Drawing for the job (mm, zero at the part's lowest x, y, z). A direction names the side the tool comes from. Give positions to 0.01 mm unless a question says otherwise; leave off trailing zeros. Order: outer loops, then holes, each group sorted by start corner. A loop starts at its lowest first (then second) coordinate and runs counter-clockwise, first axis right, second up. Notation, with made-up numbers: (69.25, -33.5) - (104.25, -33.5) arc R23 cw to (104.25, -22.5) - close; hole circle Ø9 at (-17.5, 41.5). An arc over 180 degrees is marked (long way). Use a Markdown table: item, result. Add a question column.
(1) Which spindle directions (+Z, -Z, +X, -X, +Y, -Y) get a long thin tool onto all of the face, cutting with end or side? Do the marked faces 1, 2, 3 and 4. Say none if no direction does.
(2) Wall check: line 1 (X direction, y = 39.5, z = 6); line 2 (Y direction, x = 3.75, z = 21); line 3 (Z direction, x = 10.75, y = 27). Give the ranges that are in metal, low to high.
(3) Flat gauge pins, fed straight in: pin 1 (9.5 mm diameter, centred on y = 12.5, z = 17.5, fed in from +X); pin 2 (8 mm diameter, centred on x = 20.5, y = 33, fed in from +Z); pin 3 (3 mm diameter, centred on y = 36, z = 21, fed in from -X). Where does each tip first touch, or does it go through?
(4) Slice it at C-C (y = 4). Write the cut outline in (x, z).
(5) Slice it at B-B (z = 23). Write the cut outline in (x, y), then the cut area to 3 significant figures.
(6) Slice it at D-D (x = 22.25). Write the cut outline in (y, z).
(7) Slice it at A-A (x = 14). Write the cut outline in (y, z).
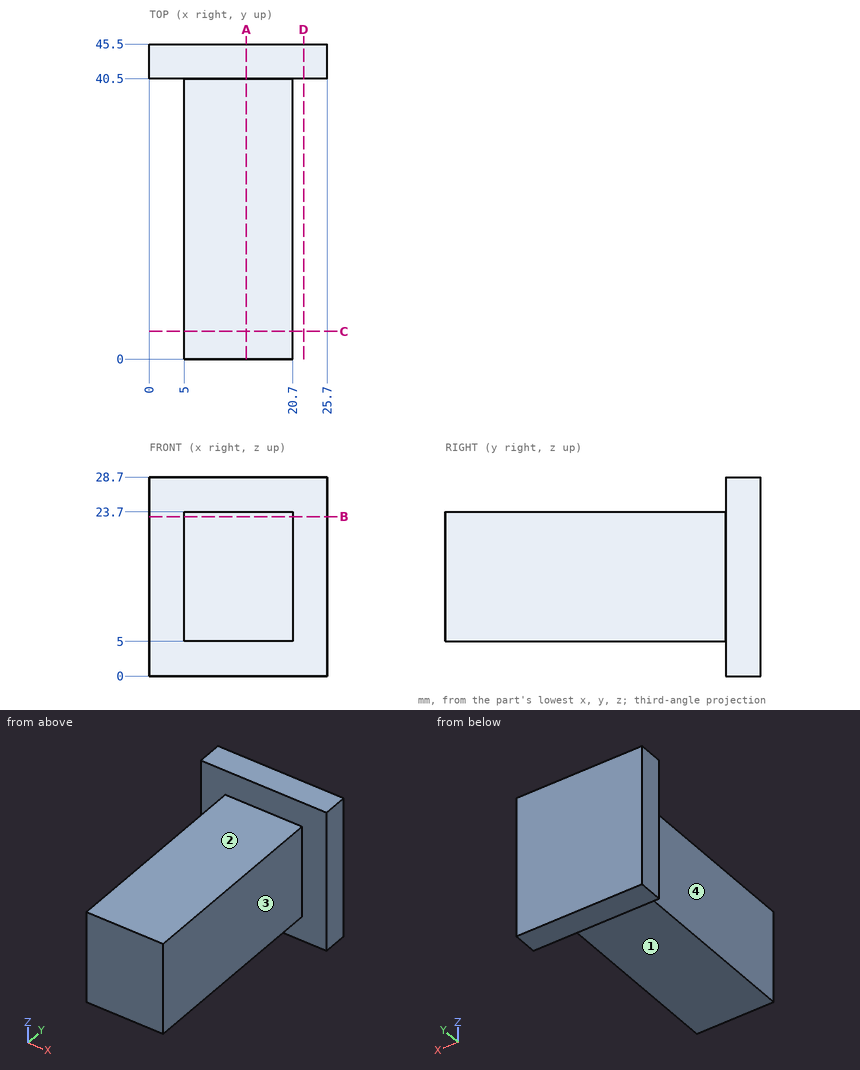
Solution:
| question | item | result |
|---|---|---|
| 1 | face 1 | -Z, +X, -X, -Y |
| 1 | face 2 | +Z, +X, -X, -Y |
| 1 | face 3 | +Z, -Z, +X, -Y |
| 1 | face 4 | +Z, -Z, -X, -Y |
| 2 | line 1 | 5 to 20.7 |
| 2 | line 2 | 40.5 to 45.5 |
| 2 | line 3 | 5 to 23.7 |
| 3 | pin 1 | x = 20.7 |
| 3 | pin 2 | z = 23.7 |
| 3 | pin 3 | x = 5 |
| 4 | outline | (5, 5) - (20.7, 5) - (20.7, 23.7) - (5, 23.7) - close |
| 5 | outline | (0, 40.5) - (5, 40.5) - (5, 0) - (20.7, 0) - (20.7, 40.5) - (25.7, 40.5) - (25.7, 45.5) - (0, 45.5) - close |
| 5 | area | 764 mm2 |
| 6 | outline | (40.5, 0) - (45.5, 0) - (45.5, 28.7) - (40.5, 28.7) - close |
| 7 | outline | (0, 5) - (40.5, 5) - (40.5, 0) - (45.5, 0) - (45.5, 28.7) - (40.5, 28.7) - (40.5, 23.7) - (0, 23.7) - close |
